from build123d import *

# Parameters (mm, degrees)
SKETCH1_W           = 304.8
SKETCH1_H           = 177.8
BOSS_EXTRUDE1_DEPTH = 19.05
SKETCH2_R           = 2.5527
SKETCH2_R_2         = 1.63195
SKETCH2_R_3         = 9.525
CUT_EXTRUDE1_DEPTH  = 178.459495379
SKETCH10_R          = 2.5527
CUT_EXTRUDE2_DEPTH  = 178.459495379


with BuildPart() as part:
    # Sketch1 → Boss-Extrude1 (new body)
    with BuildSketch(Plane.XY):
        Rectangle(SKETCH1_W, SKETCH1_H)
    extrude(amount=-BOSS_EXTRUDE1_DEPTH)

    # Sketch2 → Cut-Extrude1 (cut, through all)
    with BuildSketch(Plane.XY):
        with Locations((-104.248655176, -12.758541966)):
            Circle(SKETCH2_R)
        with Locations((-46.793240461, -46.174477312)):
            Circle(SKETCH2_R)
        with Locations((18.05555, 16.7132)):
            Circle(SKETCH2_R)
        with Locations((-35.851762373, 53.135528594)):
            Circle(SKETCH2_R)
        with Locations((-47.693929175, -72.1868)):
            Circle(SKETCH2_R)
        with Locations((49.80555, 48.4632)):
            Circle(SKETCH2_R)
        with Locations((81.55555, 16.7132)):
            Circle(SKETCH2_R)
        with Locations((49.80555, -15.0368)):
            Circle(SKETCH2_R)
        with Locations((-46.793240461, -14.002181532)):
            Circle(SKETCH2_R)
        with Locations((49.80555, 73.8632)):
            Circle(SKETCH2_R_2)
        with Locations((145.05555, -72.1868)):
            Circle(SKETCH2_R)
        with Locations((-0.418847989, -10.556423149)):
            Circle(SKETCH2_R_2)
        with Locations((97.735572958, -14.412920851)):
            Circle(SKETCH2_R_2)
        with Locations((49.80555, 16.7132)):
            Circle(SKETCH2_R_3)
    extrude(amount=-CUT_EXTRUDE1_DEPTH, mode=Mode.SUBTRACT)

    # Sketch10 → Cut-Extrude2 (cut, through all)
    with BuildSketch(Plane.XY):
        with Locations((-12.473887774, 0)):
            Circle(SKETCH10_R)
        with Locations((31.026112348, -43.500000122)):
            Circle(SKETCH10_R)
        with Locations((74.52611247, 0)):
            Circle(SKETCH10_R)
        with Locations((31.026112348, 43.500000122)):
            Circle(SKETCH10_R)
        with Locations((31.026112348, 22.225)):
            Circle(SKETCH10_R)
        with Locations((31.026112348, -22.225)):
            Circle(SKETCH10_R)
    extrude(amount=-CUT_EXTRUDE2_DEPTH, mode=Mode.SUBTRACT)


solid = part.part
Verification items for the finished model (mm, model axes). Give positions to 0.01 mm unless a question says otherwise; leave off trailing zeros. Loops run counter-clockwise (first coordinate to the right, second up) from the corner with the lowest first, then second, coordinate; pieces in that order, holes last.
1) Sectioned sample at A-A, the plane x = 56.5. Enter the section's corners in (y, z).
2) Thickness scan on line 1 along Y through (x, z) = (32, -0.75); line 2 along X through (y, z) = (52.5, -7); line 3 along X through (y, z) = (-13, -10.75). Record the ranges inside material, lowest first.
3) Depth check by flat-ended pin: pin 1 Ø6 at (x, y) = (81.56, 16.71) entering from -Z. Enter the tip coordinate at first touch or a pass-through.
4) Draft check along Y on faces 1 (the flat face through (-2, 88.9, -9)), 2 (the flat face through (-2, -88.9, -9)), 3 (the flat face through (-2, 1, -19.05)), 4 (the cylindrical face through (58.89, 19.57, -9.39)). Enter one of: pulls with the +Y half, pulls with the -Y half, needs draft (parallel to the pull), parting line crosses it, or undercut.
Answers:
1. outline: (-88.9, -19.05) - (9.94, -19.05) - (9.94, 0) - (-88.9, 0) - close; (23.49, -19.05) - (88.9, -19.05) - (88.9, 0) - (23.49, 0) - close
2. line 1: y = -88.9 to -45.86, -41.14 to -24.58, -19.87 to 19.87, 24.58 to 41.14, 45.86 to 88.9
2. line 2: x = -152.4 to -38.32, -33.38 to 152.4
2. line 3: x = -152.4 to -106.79, -101.71 to -49.14, -44.45 to 48.27, 51.34 to 96.92, 98.55 to 152.4
3. pin 1: stops at z = -19.05
4. face 1: pulls with the +Y half
4. face 2: pulls with the -Y half
4. face 3: needs draft
4. face 4: undercut
